from build123d import *

# Parameters (mm, degrees)
F1_DEPTH = 25.4
F0_W     = 25.4
F0_H     = 12.7
F2_DEPTH = 38.1
F3_DEPTH = 12.7
F5_DEPTH = 12.7
F7_DEPTH = 12.7


with BuildPart() as f1:
    # F0 (on Right) → F1 (new body)
    with BuildSketch(Plane.YZ):
        Polygon((25.4, 12.7), (25.4, 0), (127, 0), (127, 38.1), (107.95, 57.15), (63.5, 57.15), (19.05, 57.15), (0, 57.15), (0, 12.7), align=None)
    extrude(amount=F1_DEPTH)

    # F0 (on Right) → F2 (join)
    with BuildSketch(Plane.YZ):
        with Locations((12.7, 6.35)):
            Rectangle(F0_W, F0_H)
    extrude(amount=F2_DEPTH)

    # F0 (on Right) → F3 (join)
    with BuildSketch(Plane.YZ):
        Polygon((19.05, 76.2), (19.05, 57.15), (63.5, 57.15), (44.45, 76.2), align=None)
    extrude(amount=F3_DEPTH)

    # F4 (on face) → F5 (cut)
    with BuildSketch(Plane.XY.offset(12.7)):
        Polygon((25.4, 25.4), (38.1, 12.7), (38.1, 25.4), align=None)
    extrude(amount=-F5_DEPTH, mode=Mode.SUBTRACT)

    # F6 (on face) → F7 (cut)
    with BuildSketch(Plane.YZ.offset(12.7)):
        Polygon((43.3805931771, 73.66), (21.59, 73.66), (21.59, 59.69), (57.3505931771, 59.69), (52.1702965885, 64.8702965885), align=None)
    extrude(amount=-F7_DEPTH, mode=Mode.SUBTRACT)

    # F8: F1 across plane


with BuildPart() as f1_1:
    add(f1.part)
    add(f1.part.mirror(Plane.YZ))


solid = f1_1.part
Work out the finished part from the listing and answer in its coordinate system (mm). A direction names the side the tool comes from. Round coordinates to 2 decimals unless told otherwise and drop trailing zeros. Loops run counter-clockwise (first coordinate to the right, second up) from the corner with the lowest first, then second, coordinate; pieces in that order, holes last. Notation, with made-up numbers: (-31, 7) - (-19, 7) arc R25 cw to (-19, 30) - close; hole circle Ø10 at (-8, 45.5). An arc over 180 degrees is marked (long way). Use one line per item in the form item = value. Start each with the question number.
(1) Consider line 1 (Z direction, x = -16, y = 18.5); line 2 (X direction, y = 59, z = 32.5); line 3 (Y direction, x = -4, z = 70.5). Determine where each line is inside the solid, lowest interval first.
(2) Find section D-D on z = 9. Determine the outline of the cut face in (x, y), and give its area (3 significant figures).
(3) Determine the mould class of faces 1 (the face through (0, 127, 19)), 2 (the face through (32, 10, 12.7)), 3 (the face through (0, 21.59, 67)), 4 (the face through (0, 39, 59.69)) for opening direction Z: +Z half, -Z half, draft (parallel to the pull), parting line (faces both ways), or undercut.
(4) Find section C-C on y = 37. Determine the outline of the cut face in (x, z), and give its area (3 significant figures).
(5) Flat-ended cylindrical pins translate along their axes: P1, Ø17.5, axis at x = 0.5, y = 28, coming from the -Z side; P2, Ø21, axis at y = 50, z = 71.5, coming from the -X side; P3, Ø17, axis at y = 73, z = 32.5, coming from the +X side; P4, Ø10, axis at x = -29, z = 56, coming from the +Y side. Find the tip coordinate at first contact, or state that the pin passes through.
(6) Find section A-A on x = -7.5. Determine the outline of the cut face in (y, z).
(7) Find section B-B on z = 68.5. Determine the outline of the cut face in (x, y), and give its area (3 significant figures).
(8) Which of the six approach directions +Z, -Z, +X, -X, +Y, -Y give full straight-line access (tool end or side, diameter ignored) to faces 5 (the face through (-32, 10, 12.7)), 6 (the face through (-25.4, 63, 29)), 7 (the face through (12.7, 35, 59)), 8 (the face through (0, 19.05, 67))?
Answer list:
q1.line_1 = 0 to 57.15
q1.line_2 = -25.4 to 25.4
q1.line_3 = 19.05 to 21.59, 46.54 to 50.15
q2.outline = (-38.1, 0) - (38.1, 0) - (38.1, 12.7) - (25.4, 25.4) - (25.4, 127) - (-25.4, 127) - (-25.4, 25.4) - (-38.1, 12.7) - close
q2.area = 6,940 mm^2
q3.face_1 = draft
q3.face_2 = +Z half
q3.face_3 = undercut
q3.face_4 = undercut
q4.outline = (-25.4, 0) - (25.4, 0) - (25.4, 57.15) - (12.7, 57.15) - (12.7, 59.69) - (-12.7, 59.69) - (-12.7, 57.15) - (-25.4, 57.15) - close; (-12.7, 73.66) - (12.7, 73.66) - (12.7, 76.2) - (-12.7, 76.2) - close
q4.area = 3,030 mm^2
q5.P1 = 0
q5.P2 = -12.7
q5.P3 = 25.4
q5.P4 = 112.57
q6.outline = (0, 0) - (127, 0) - (127, 38.1) - (107.95, 57.15) - (63.5, 57.15) - (44.45, 76.2) - (19.05, 76.2) - (19.05, 57.15) - (0, 57.15) - close; hole (21.59, 59.69) - (57.35, 59.69) - (43.38, 73.66) - (21.59, 73.66) - close
q7.outline = (-12.7, 19.05) - (12.7, 19.05) - (12.7, 21.59) - (-12.7, 21.59) - close; (-12.7, 48.54) - (12.7, 48.54) - (12.7, 52.15) - (-12.7, 52.15) - close
q7.area = 156 mm^2
q8.face_5 = +Z, -X, +Y, -Y
q8.face_6 = +Z, -X, +Y
q8.face_7 = +Z, +X, +Y, -Y
q8.face_8 = +Z, +X, -X, -Y
